Input: dimensioned drawing with shaded views. Units: mm. Origin: part minimum x, y, z. Give positions to 0.01 mm unless a question says otherwise; leave off trailing zeros. Order: outer loops, then holes, each group sorted by start corner. A loop starts at its lowest first (then second) coordinate and runs counter-clockwise, first axis right, second up. Notation, with made-up numbers: (31.5, 31.25) -> (65.5, 31.25) arc R14 cw to (65.5, 58.25) -> close; hole circle Ø9 at (30.5, 1.5). An arc over 180 degrees is marked (long way). One line per question, with ' | ' between items. Start each with the question number.
(1) Section A-A (x = 6.75). Return loops of the section in (y, z).
(2) Section B-B (z = 16.25). Return loops of the section in (x, y).
(3) Ray query, L1, parallel to Z at x = 3.75, y = 4.75; L2, parallel to Z at x = 4, y = 1.75; L3, parallel to Y at x = 5, z = 18.5. Return the intervals inside material, ascending.
(4) Section C-C (y = 3). Return loops of the section in (x, z), then the cut area to 3 significant figures.
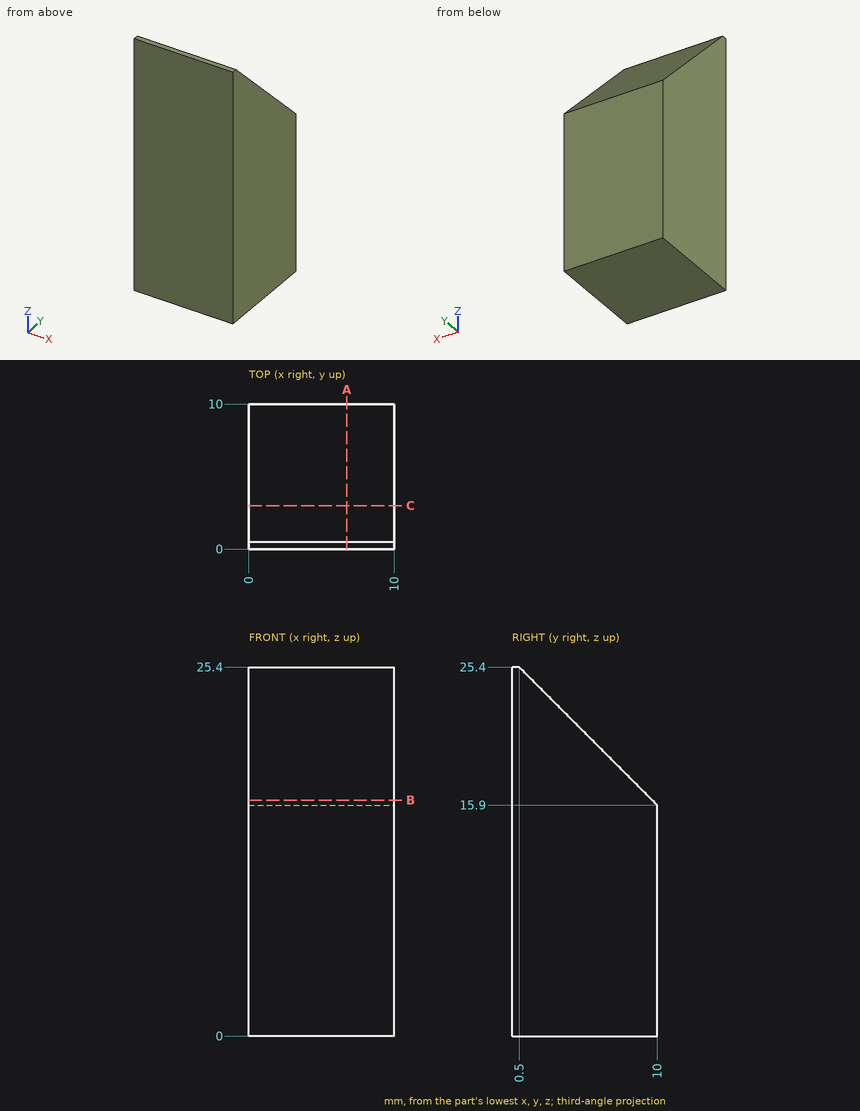
Response:
1) outline: (0, 0) -> (10, 0) -> (10, 15.9) -> (0.5, 25.4) -> (0, 25.4) -> close
2) outline: (0, 0) -> (10, 0) -> (10, 9.65) -> (0, 9.65) -> close
3) L1: z = 0 to 21.15 | L2: z = 0 to 24.15 | L3: y = 0 to 7.4
4) outline: (0, 0) -> (10, 0) -> (10, 22.9) -> (0, 22.9) -> close | area: 229 mm^2
